Verification items for the finished model (mm, model axes). A direction names the side the tool comes from. Round coordinates to 2 decimals unless told otherwise and drop trailing zeros. Order: outer loops, then holes, each group sorted by start corner. A loop starts at its lowest first (then second) coordinate and runs counter-clockwise, first axis right, second up. Notation, with made-up numbers: M -35.5,36.5 L -16.5,36.5 A36 cw -16.5,71.5 Z; hole C 64,-11.75 d6. An arc over 180 degrees is marked long. Return JSON: item names as keys, results as strings. Group by question number.
Autodesk Inventor part; units mm, degrees
ref_plane "YZ Plane" through (0, 0, 0) normal (1, 0, 0) x (0, 1, 0)
ref_plane "XZ Plane" through (0, 0, 0) normal (0, 1, 0) x (-1, 0, 0)
ref_plane "XY Plane" through (0, 0, 0) normal (0, 0, 1) x (1, 0, 0)
sketch "Sketch1" plane through (0, 0, 0) normal (0, 1, 0) x (-1, 0, 0)
  line L0 (0, 0) -> (13.6144, 0)
  circle A0 centre (0, 0) radius 17.78
  dimension "d0" = 13.6144
  dimension "d1" = 35.56
extrude "Extrusion1" add sketch "Sketch1" along normal blind 19.05
sketch "Sketch3" plane through (0, 19.05, 0) normal (0, 1, 0) x (1, 0, 0)
  line L0 (0, 0) -> (0, 13.6144)
  line L1 (0, 0) -> (13.6144, 0) construction
  dimension "d4" = 13.6144
  dimension "d5" = 90
hole "Hole1" at (0, 19.05, -13.6144) direction (0, -1, 0) diameter 4.9022 end through all counterbore diameter 7.239 counterbore depth 5.08
sketch "Sketch4" plane through (0, 0, 0) normal (0, -1, 0) x (1, 0, 0)
  circle A0 centre (0, -13.6144) radius 2.4511
  line L0 (0, 0) -> (0, -13.6144)
hole "Hole2" at (0, 0, -13.6144) direction (0, 1, 0) diameter 4.9022 depth 6.35 counterbore diameter 6.5532 counterbore depth 1.6002
pattern_circular "Circular Pattern1" count 3 over 360 about axis through (0, 0, 0) along (0, 1, 0) of "Hole1", "Hole2"
sketch "Sketch6" plane through (0, 19.05, 0) normal (0, 1, 0) x (1, 0, 0)
  point P0 (0, 0)
  point P1 (0, 0)
hole "Hole3" at (0, 19.05, 0) direction (0, -1, 0) diameter 6.35 end through all
sketch "Sketch10" plane through (0, 0, 0) normal (0, -1, 0) x (1, 0, 0)
  line L0 (7.9434, 13.6879) -> (-4.7505, 14.0829)
  line L1 (-4.7505, 14.0829) -> (-4.8208, 11.8209)
  line L2 (-4.8208, 11.8209) -> (7.873, 11.426)
  line L3 (7.873, 11.426) -> (7.9434, 13.6879)
  line L4 (11.4066, 0) -> (4.9497, -10.9361)
  line L5 (4.9497, -10.9361) -> (7.1371, -12.2276)
  line L6 (7.1371, -12.2276) -> (13.2977, -1.0415)
  line L7 (13.2977, -1.0415) -> (11.4066, 0)
  point P0 (0, 0)
  dimension "d38" = 12.7
  dimension "d39" = 12.7
extrude "Extrusion2" cut sketch "Sketch10" against normal blind 12.7
properties part number "table"
1. Go/stop test with flat-tipped pins: pin 1 (6 mm diameter, centred on x = 0, z = -13.61, fed in from -Y); pin 2 (2 mm diameter, centred on x = -1.5, z = -15, fed in from +Y); pin 3 (2 mm diameter, centred on x = -12.5, y = 7.5, fed in from +Z); pin 4 (4 mm diameter, centred on x = 0, z = -13.61, fed in from +Y). Record where each tip stops, or that it passes through.
2. Thickness scan on line 1 along Z through (x, y) = (0, 0.4) (3 decimals); line 2 along X through (y, z) = (12.25, 5); line 3 along X through (y, z) = (13.75, -14.5). Record the ranges inside material, lowest first. Write a range as from..to.
3. Access from +Z, -Z, +X, -X, +Y, -Y to the whole of each face (thin tool, end or side, straight path). Record for faces 1 (the face through (-14, 1.6, 5)), 2 (the face through (9, 13.97, 6)), 3 (the face through (3.1, 9.39, -0.69)).
4. Cross-section at A-A (x = -10.5). Enter the section's corners in (y, z), plus the area to 3 significant figures.
5. Cross-section at C-C (y = 6.5). Give the number of separate pieces and of enclosed holes in the cut face, plus the area to 3 significant figures.
6. Cross-section at B-B (z = 1). Enter the section's corners in (x, y).
7. Draft check along Z on faces 4 (the face through (0, 0, -4)), 5 (the face through (1, 13.97, -11)). Enter one of: +Z half, -Z half, draft (parallel to the pull), parting line (faces both ways), or undercut.
Computed:
{
 "1": {"pin 1": "stops at y = 1.6", "pin 2": "stops at y = 13.97", "pin 3": "stops at z = 13.56", "pin 4": "passes through"},
 "2": {"line 1": "z = -17.78..-16.891, -10.338..-3.175, 3.175..11.671, 13.935..17.78", "line 2": "x = -17.06..-13.45, -10.13..10.13, 13.45..17.06", "line 3": "x = -10.29..-2.29, 2.29..10.29"},
 "3": {"face 1": "-Y", "face 2": "+Y", "face 3": "+Y, -Y"},
 "4": {"outline": "M 0,-14.35 L 19.05,-14.35 L 19.05,3.43 L 13.97,3.43 L 13.97,4.72 L 1.6,4.72 L 1.6,3.8 L 0,3.8 Z; M 0,9.82 L 1.6,9.82 L 1.6,8.89 L 13.97,8.89 L 13.97,10.19 L 19.05,10.19 L 19.05,14.35 L 0,14.35 Z", "area": "451 mm²"},
 "5": {"separate pieces": "1", "enclosed holes": "6", "area": "846 mm²"},
 "6": {"outline": "M -17.75,0 L -3.01,0 L -3.01,19.05 L -17.75,19.05 Z; M 3.01,0 L 17.75,0 L 17.75,19.05 L 3.01,19.05 Z"},
 "7": {"face 4": "draft", "face 5": "undercut"}
}
